Source: CAD feature listing. Evaluate the final solid. Frame: model axes, mm. A direction names the side the tool comes from. Give positions to 0.01 mm unless a question says otherwise; leave off trailing zeros. Loops run counter-clockwise (first coordinate to the right, second up) from the corner with the lowest first, then second, coordinate; pieces in that order, holes last.
from build123d import *

# Parameters (mm, degrees)
SKETCH1_R           = 3.6
BOSS_EXTRUDE1_DEPTH = 2
SKETCH2_W           = 3
SKETCH2_H           = 3
BOSS_EXTRUDE2_DEPTH = 20
SKETCH3_W           = 1.5
SKETCH3_H           = 3.039979134
CUT_EXTRUDE1_DEPTH  = 3
SKETCH4_W           = 3.039979134
SKETCH4_H           = 13.71909755
SKETCH4_W_2         = 1.039979134
SKETCH4_H_2         = 11.71909755
BOSS_EXTRUDE3_DEPTH = 1.5


with BuildPart() as part:
    # Sketch1 → Boss-Extrude1 (new body)
    with BuildSketch(Plane.XY):
        Circle(SKETCH1_R)
    extrude(amount=BOSS_EXTRUDE1_DEPTH)

    # Sketch2 → Boss-Extrude2 (add)
    with BuildSketch(Plane.XY.offset(2)):
        Rectangle(SKETCH2_W, SKETCH2_H)
    extrude(amount=BOSS_EXTRUDE2_DEPTH)

    # Sketch3 → Cut-Extrude1 (cut)
    with BuildSketch(Plane(origin=(0, 1.5, 0), x_dir=(1, 0, 0), z_dir=(0, 1, 0))):
        with Locations((-0.75, -20.480010433)):
            Rectangle(SKETCH3_W, SKETCH3_H)
    extrude(amount=-CUT_EXTRUDE1_DEPTH, mode=Mode.SUBTRACT)

    # Sketch4 → Boss-Extrude3 (add)
    with BuildSketch(Plane.ZY):
        with Locations((20.480010433, 0.024038237)):
            Rectangle(SKETCH4_W, SKETCH4_H)
        with Locations((20.480010433, 0.024038237)):
            Rectangle(SKETCH4_W_2, SKETCH4_H_2, mode=Mode.SUBTRACT)
    extrude(amount=BOSS_EXTRUDE3_DEPTH)


solid = part.part
1) Cut plane C-C (x = -1). Return loops of the section in (y, z), and give its area (3 significant figures).
Checks:
outline: (-6.84, 18.96) - (-1.5, 18.96) - (-1.5, 2) - (-3.46, 2) - (-3.46, 0) - (3.46, 0) - (3.46, 2) - (1.5, 2) - (1.5, 18.96) - (6.88, 18.96) - (6.88, 22) - (-6.84, 22) - close; hole (-5.84, 19.96) - (5.88, 19.96) - (5.88, 21) - (-5.84, 21) - close
area: 94.2 mm2
2) Pull-direction query (Z, two-part tool) for faces 1 (the flat face through (0, 0, 0)), 2 (the flat face through (0, -4.1, 19.8)), 3 (the flat face through (-0.7, -5.836, 20.5)); classes: released by +Z, released by -Z, zero draft, split by the parting line, or undercut.
Checks:
face 1: released by -Z
face 2: zero draft
face 3: undercut
3) Ray query, probe 1 along Z at (x, y) = (-1, -3); probe 2 along Z at (x, y) = (-0.5, -5); probe 3 along Z at (x, y) = (1.75, 0.25). Return the intervals inside material, ascending.
Checks:
probe 1: z = 0 to 2, 18.96 to 19.96, 21 to 22
probe 2: z = 18.96 to 19.96, 21 to 22
probe 3: z = 0 to 2
4) Contact query for flat-ended pins moving along their axis: P1, Ø1.5, axis at y = -2.5, z = 16.5, coming from the +X side; P2, Ø4, axis at y = 0, z = 8, coming from the -X side; P3, Ø1.5, axis at y = 3.5, z = 20, coming from the +X side; P4, Ø2, axis at x = 1, z = 16.5, coming from the +Y side. Output: stop coordinate, or through.
Checks:
P1: passes through
P2: stops at x = -1.5
P3: stops at x = 0
P4: stops at y = 1.5
5) Cut plane D-D (x = 1.25). Return loops of the section in (y, z), and give its area (3 significant figures).
Checks:
outline: (-3.38, 0) - (3.38, 0) - (3.38, 2) - (1.5, 2) - (1.5, 22) - (-1.5, 22) - (-1.5, 2) - (-3.38, 2) - close
area: 73.5 mm2
6) Cut plane A-A (y = 5.5). Return loops of the section in (x, z), and give its area (3 significant figures).
Checks:
outline: (-1.5, 18.96) - (0, 18.96) - (0, 19.96) - (-1.5, 19.96) - close; (-1.5, 21) - (0, 21) - (0, 22) - (-1.5, 22) - close
area: 3.00 mm2
7) Reachability of faces 4 (the flat face through (-1.5, 0, 13)), 5 (the flat face through (-1, 0, 21)), 6 (the flat face through (-1, 4, 18.96)), 7 (the flat face through (-0.7, 5.884, 20.5)), 8 (the flat face through (-1, -4, 18.96)) from +Z, -Z, +X, -X, +Y, -Y: full face, straight path, thin tool, end or side. Return the list, or none.
Checks:
face 4: +Z, -X, +Y, -Y
face 5: -X
face 6: +X, -X, +Y
face 7: +X, -X
face 8: +X, -X, -Y
8) Cut plane B-B (y = 0). Return loops of the section in (x, z).
Checks:
outline: (-3.6, 0) - (3.6, 0) - (3.6, 2) - (1.5, 2) - (1.5, 22) - (-1.5, 22) - (-1.5, 21) - (0, 21) - (0, 19.96) - (-1.5, 19.96) - (-1.5, 2) - (-3.6, 2) - close
